Input: part model. Units: mm. Frame: model coordinates. Face numbers are marked on the shaded views. A direction names the side the tool comes from. Round coordinates to 2 decimals unless told otherwise and drop trailing zeros. Loops run counter-clockwise (first coordinate to the right, second up) from the corner with the lowest first, then second, coordinate; pieces in that order, holes last.
(1) First-contact query: pin 1 Ø0.6 at (x, y) = (-45, 4) entering from +Z; pin 2 Ø10 at (x, z) = (-2, -8) entering from -Y; pin 3 Ø2 at (x, y) = (-5, -12) entering from -Z (3 decimals). Flat tips, straight axial feed; report the tip coordinate or a pass-through.
(2) Cut plane C-C, the plane x = 8.15. Give the number of separate pieces and of enclosed holes in the cut face, and give its area (3 significant figures).
(3) Cut plane B-B, the plane z = -10. Output: boundary loops of the cut face in (x, y), and give its area (3 significant figures).
(4) Line query: line 1 (Z direction, x = 8.15, y = 1.2) (3 decimals); line 2 (Z direction, x = 16, y = -12.5) (3 decimals); line 3 (Y direction, x = 27, z = -32). Output: solid intervals per line, ascending.
(5) Access query for the marked faces 4 and 5. Directions: +Z, -Z, +X, -X, +Y, -Y. A direction counts if a zero-diameter tool reaches every point of the face in a straight line with its end or side. Return the directions, or none.
(6) Cut plane D-D, the plane x = -14. Output: boundary loops of the cut face in (y, z) (3 decimals), and give its area (3 significant figures).
(7) Draft query along Z for the marked faces 1, 2 and 3. Return one class per face: released by +Z, released by -Z, zero draft, split by the parting line, or undercut.
(8) Cut plane A-A, the plane y = -34. Output: boundary loops of the cut face in (x, z) (3 decimals).
from build123d import *

# Parameters (mm, degrees)
SKETCH1_W                = 40
SKETCH1_H                = 40
BOSS_EXTRUDE1_DEPTH      = 2
SKETCH10_W               = 40
SKETCH10_H               = 2
BOSS_EXTRUDE4_DEPTH      = 4
SKETCH11_W               = 40
SKETCH11_H               = 40
BOSS_EXTRUDE5_DEPTH      = 2
M3_CLEARANCE_HOLE1_D     = 3.4
SKETCH5_W                = 40
SKETCH5_H                = 2
BOSS_EXTRUDE2_DEPTH      = 48
SKETCH6_W                = 2
SKETCH6_H                = 40
BOSS_EXTRUDE3_DEPTH      = 6
SKETCH7_W                = 2
SKETCH7_H                = 28
CUT_EXTRUDE1_DEPTH       = 6
M3_CLEARANCE_HOLE2_D     = 3.4
M3_CLEARANCE_HOLE2_DEPTH = 2
M3_CLEARANCE_HOLE2_TIP   = 1.021463052
SKETCH12_W               = 36
SKETCH12_H               = 4
CUT_EXTRUDE2_DEPTH       = 63.992062992
EXTRUDE_THIN1_REACH      = 64.769
SKETCH13_R               = 3.7
SKETCH13_R_2             = 1.7
SKETCH14_W               = 40
SKETCH14_H               = 2
BOSS_EXTRUDE6_DEPTH      = 44.465
M3_CLEARANCE_HOLE3_D     = 3.4
SKETCH19_W               = 40
SKETCH19_H               = 2
BOSS_EXTRUDE7_DEPTH      = 44.465
SKETCH20_R               = 1.7
CUT_EXTRUDE3_DEPTH       = 98.479927293
CUT_EXTRUDE4_DEPTH       = 98.479927293
SKETCH24_W               = 44.465
SKETCH24_H               = 2
BOSS_EXTRUDE9_DEPTH      = 40
SKETCH22_W               = 40
SKETCH22_H               = 3
BOSS_EXTRUDE8_DEPTH      = 60
FILLET1_R                = 2
CUT_EXTRUDE5_REACH       = 122.894
SKETCH23_R               = 12.5
FILLET1_OF_MIRROR1_R     = 2


with BuildPart() as part:
    # Sketch1 → Boss-Extrude1 (new body)
    with BuildSketch(Plane(origin=(0, 0, 0), x_dir=(1, 0, 0), z_dir=(0, 1, 0))):
        with Locations((20, 20)):
            Rectangle(SKETCH1_W, SKETCH1_H)
    extrude(amount=BOSS_EXTRUDE1_DEPTH)

    # Sketch10 → Boss-Extrude4 (add)
    with BuildSketch(Plane(origin=(0, 2, 0), x_dir=(1, 0, 0), z_dir=(0, 1, 0))):
        with Locations((20, 1)):
            Rectangle(SKETCH10_W, SKETCH10_H)
        with Locations((20, 39)):
            Rectangle(SKETCH10_W, SKETCH10_H)
    extrude(amount=BOSS_EXTRUDE4_DEPTH)

    # Sketch11 → Boss-Extrude5 (add)
    with BuildSketch(Plane(origin=(0, 6, 0), x_dir=(1, 0, 0), z_dir=(0, 1, 0))):
        with Locations((20, 20)):
            Rectangle(SKETCH11_W, SKETCH11_H)
    extrude(amount=BOSS_EXTRUDE5_DEPTH)

    # M3 Clearance Hole1 (through all)
    with Locations(Plane.XZ):
        with Locations((8.15, -30), (8.15, -10), (31.85, -20)):
            Hole(M3_CLEARANCE_HOLE1_D / 2)

    # Sketch5 → Boss-Extrude2 (add)
    with BuildSketch(Plane(origin=(0, 0, 0), x_dir=(0, 0, -1), z_dir=(1, 0, 0))):
        with Locations((20, 7)):
            Rectangle(SKETCH5_W, SKETCH5_H)
    extrude(amount=-BOSS_EXTRUDE2_DEPTH)

    # Sketch6 → Boss-Extrude3 (add)
    with BuildSketch(Plane(origin=(-6, 6, 0), x_dir=(-1, 0, 0), z_dir=(0, 1, 0))):
        with Locations((39, -20)):
            Rectangle(SKETCH6_W, SKETCH6_H)
    extrude(amount=-BOSS_EXTRUDE3_DEPTH)

    # Sketch7 → Cut-Extrude1 (cut)
    with BuildSketch(Plane(origin=(46, 0, 0), x_dir=(-1, 0, 0), z_dir=(0, 1, 0))):
        with Locations((91, -20)):
            Rectangle(SKETCH7_W, SKETCH7_H)
    extrude(amount=CUT_EXTRUDE1_DEPTH, mode=Mode.SUBTRACT)

    # M3 Clearance Hole2
    with Locations(Plane(origin=(-46, 0, 0), x_dir=(0, 0, -1), z_dir=(-1, 0, 0))):
        with Locations((3, -3), (37, -3)):
            Hole(M3_CLEARANCE_HOLE2_D / 2, depth=M3_CLEARANCE_HOLE2_DEPTH)
            with Locations((0, 0, -(M3_CLEARANCE_HOLE2_DEPTH + M3_CLEARANCE_HOLE2_TIP / 2))):  # 118° drill point
                Cone(0, M3_CLEARANCE_HOLE2_D / 2, M3_CLEARANCE_HOLE2_TIP, mode=Mode.SUBTRACT)

    # Sketch12 → Cut-Extrude2 (cut, through all)
    with BuildSketch(Plane(origin=(0, 0, -40), x_dir=(-1, 0, 0), z_dir=(0, 0, -1))):
        with Locations((-20, 4)):
            Rectangle(SKETCH12_W, SKETCH12_H)
    extrude(amount=-CUT_EXTRUDE2_DEPTH, mode=Mode.SUBTRACT)

    # Sketch13 → Extrude-Thin1 (add, up to next)
    with BuildSketch(Plane(origin=(0, 2, 0), x_dir=(1, 0, 0), z_dir=(0, 1, 0)), mode=Mode.PRIVATE) as extrude_thin1_sk1:
        with Locations((31.85, 20)):
            Circle(SKETCH13_R)
        with Locations((31.85, 20)):
            Circle(SKETCH13_R_2, mode=Mode.SUBTRACT)
    extrude_thin1_tool1 = extrude(extrude_thin1_sk1.sketch, amount=EXTRUDE_THIN1_REACH, mode=Mode.PRIVATE) - part.part
    # Sketch13 → Extrude-Thin1 (add, up to next)
    with BuildSketch(Plane(origin=(0, 2, 0), x_dir=(1, 0, 0), z_dir=(0, 1, 0)), mode=Mode.PRIVATE) as extrude_thin1_sk2:
        with Locations((8.15, 10)):
            Circle(SKETCH13_R)
        with Locations((8.15, 10)):
            Circle(SKETCH13_R_2, mode=Mode.SUBTRACT)
    extrude_thin1_tool2 = extrude(extrude_thin1_sk2.sketch, amount=EXTRUDE_THIN1_REACH, mode=Mode.PRIVATE) - part.part
    # Sketch13 → Extrude-Thin1 (add, up to next)
    with BuildSketch(Plane(origin=(0, 2, 0), x_dir=(1, 0, 0), z_dir=(0, 1, 0)), mode=Mode.PRIVATE) as extrude_thin1_sk3:
        with Locations((8.15, 30)):
            Circle(SKETCH13_R)
        with Locations((8.15, 30)):
            Circle(SKETCH13_R_2, mode=Mode.SUBTRACT)
    extrude_thin1_tool3 = extrude(extrude_thin1_sk3.sketch, amount=EXTRUDE_THIN1_REACH, mode=Mode.PRIVATE) - part.part
    add(extrude_thin1_tool1.solids().sort_by_distance((28.254652, 2, -20))[0])
    add(extrude_thin1_tool2.solids().sort_by_distance((4.554652, 2, -10))[0])
    add(extrude_thin1_tool3.solids().sort_by_distance((4.554652, 2, -30))[0])

    # Sketch14 → Boss-Extrude6 (add)
    with BuildSketch(Plane(origin=(0, 0, -40), x_dir=(-1, 0, 0), z_dir=(0, 0, -1))):
        with Locations((-20, 7)):
            Rectangle(SKETCH14_W, SKETCH14_H)
    extrude(amount=BOSS_EXTRUDE6_DEPTH)

    # M3 Clearance Hole3 (through all)
    with Locations(Plane(origin=(0, 8, 0), x_dir=(1, 0, 0), z_dir=(0, 1, 0))):
        with Locations((30, 45.10564971)):
            Hole(M3_CLEARANCE_HOLE3_D / 2)

    # Sketch19 → Boss-Extrude7 (add)
    with BuildSketch(Plane.XY):
        with Locations((20, 7)):
            Rectangle(SKETCH19_W, SKETCH19_H)
    extrude(amount=BOSS_EXTRUDE7_DEPTH)

    # Sketch20 → Cut-Extrude3 (cut, through all)
    with BuildSketch(Plane(origin=(0, 8, 0), x_dir=(1, 0, 0), z_dir=(0, 1, 0))):
        with Locations(Location((30, -5.10564971, 0), (0, 0, 270))):
            Circle(SKETCH20_R)
    extrude(amount=-CUT_EXTRUDE3_DEPTH, mode=Mode.SUBTRACT)

    # Sketch21 → Cut-Extrude4 (cut, through all)
    with BuildSketch(Plane(origin=(0, 8, 0), x_dir=(1, 0, 0), z_dir=(0, 1, 0))):
        Polygon((27.91, -44.465), (40, -32.375), (40, -44.465), align=None)
        Polygon((27.91, 84.465), (40, 84.465), (40, 72.375), align=None)
    extrude(amount=-CUT_EXTRUDE4_DEPTH, mode=Mode.SUBTRACT)

    # Sketch24 → Boss-Extrude9 (add)
    with BuildSketch(Plane.ZY):
        with Locations((-62.2325, 7)):
            Rectangle(SKETCH24_W, SKETCH24_H)
    boss_extrude9 = extrude(amount=BOSS_EXTRUDE9_DEPTH)

    # Sketch22 → Boss-Extrude8 (add)
    with BuildSketch(Plane.XZ.offset(-6)):
        with Locations((0, -50.965)):
            Rectangle(SKETCH22_W, SKETCH22_H)
    boss_extrude8 = extrude(amount=BOSS_EXTRUDE8_DEPTH)

    # Fillet1
    fillet1_edges = [part.edges().sort_by_distance(p)[0] for p in [
        (20, 6, -50.965),
        (0, 6, -49.465),
        (-20, 6, -50.965),
        (0, 6, -52.465),
    ]]
    fillet(fillet1_edges, radius=FILLET1_R)

    # Sketch23 → Cut-Extrude5 (cut, up to next)
    with BuildSketch(Plane(origin=(0, 0, -52.465), x_dir=(-1, 0, 0), z_dir=(0, 0, -1)), mode=Mode.PRIVATE) as cut_extrude5_sk1:
        with Locations((0, -34)):
            Circle(SKETCH23_R)
    cut_extrude5_tool1 = extrude(cut_extrude5_sk1.sketch, amount=-CUT_EXTRUDE5_REACH, mode=Mode.PRIVATE) & part.part
    cut_extrude5 = cut_extrude5_tool1.solids().sort_by_distance((0, -34, -52.465))[0]
    add(cut_extrude5, mode=Mode.SUBTRACT)

    # Mirror1: Boss-Extrude9, Boss-Extrude8, Cut-Extrude5 across plane
    add(boss_extrude9.mirror(Plane(origin=(0, 0, -20), x_dir=(1, 0, 0), z_dir=(0, 0, -1))))
    add(boss_extrude8.mirror(Plane(origin=(0, 0, -20), x_dir=(1, 0, 0), z_dir=(0, 0, -1))))
    add(cut_extrude5.mirror(Plane(origin=(0, 0, -20), x_dir=(1, 0, 0), z_dir=(0, 0, -1))), mode=Mode.SUBTRACT)

    # Fillet1 of Mirror1
    fillet1_of_mirror1_edges = [part.edges().sort_by_distance(p)[0] for p in [
        (20, 6, 10.965),
        (0, 6, 9.465),
        (-20, 6, 10.965),
        (0, 6, 12.465),
    ]]
    fillet(fillet1_of_mirror1_edges, radius=FILLET1_OF_MIRROR1_R)


solid = part.part
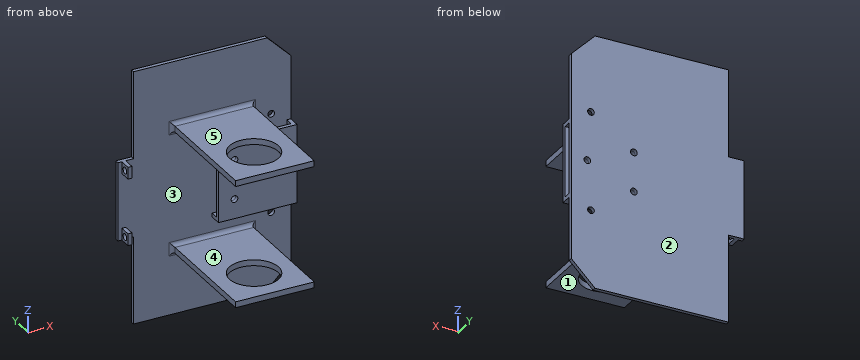
Reported:
1. pin 1: stops at z = 0
1. pin 2: stops at y = 0
1. pin 3: stops at z = -52.465
2. separate pieces: 5
2. enclosed holes: 1
2. area: 592 mm2
3. outline: (-48, 6) - (4.45, 6) - (4.45, 2) - (0, 2) - (0, 0) - (6.45, 0) - (6.45, 8) - (-48, 8) - close; (9.85, 0) - (40, 0) - (40, 2) - (11.85, 2) - (11.85, 6) - (40, 6) - (40, 8) - (9.85, 8) - close
3. area: 258 mm2
4. line 1: z = -52.465 to -49.465, -40 to -31.7, -28.3 to -11.7, -8.3 to 0, 9.465 to 12.465
4. line 2: z = -52.465 to -49.465, 9.465 to 12.465
4. line 3: y = 0 to 2, 6 to 8
5. face 4: +X, -X, -Y
5. face 5: +Z, +X, -X, -Y
6. outline: (-54, -52.465) - (4, -52.465) arc R2 cw to (6, -54.465) - (6, -84.465) - (8, -84.465) - (8, 44.465) - (6, 44.465) - (6, 14.465) arc R2 cw to (4, 12.465) - (-54, 12.465) - (-54, 9.465) - (4, 9.465) arc R2 cw to (6, 7.465) - (6, -47.465) arc R2 cw to (4, -49.465) - (-54, -49.465) - close
6. area: 621 mm2
7. face 1: released by -Z
7. face 2: zero draft
7. face 3: undercut
8. outline: (-20, -52.465) - (-12.5, -52.465) - (-12.5, -49.465) - (-20, -49.465) - close; (-20, 9.465) - (-12.5, 9.465) - (-12.5, 12.465) - (-20, 12.465) - close; (12.5, -52.465) - (20, -52.465) - (20, -49.465) - (12.5, -49.465) - close; (12.5, 9.465) - (20, 9.465) - (20, 12.465) - (12.5, 12.465) - close
